from build123d import *

# Parameters (mm, degrees)
BOSS_EXTRUDE1_DEPTH = 9
SKETCH3_R           = 17.5
SKETCH3_R_2         = 7
SKETCH3_W           = 35
SKETCH3_H           = 9
BOSS_EXTRUDE2_DEPTH = 9


with BuildPart() as part:
    # Sketch1 → Boss-Extrude1 (new body)
    with BuildSketch(Plane.XY):
        with BuildLine():
            Line((0, -20), (86, -20))
            ThreePointArc((86, -20), (106, 0), (86, 20))
            Line((86, 20), (0, 20))
            Line((0, 20), (0, -20))
        make_face()
        with BuildLine():
            Line((63, 7), (86, 7))
            ThreePointArc((86, 7), (93, 0), (86, -7))
            Line((86, -7), (63, -7))
            ThreePointArc((63, -7), (56, 0), (63, 7))
        make_face(mode=Mode.SUBTRACT)
    extrude(amount=BOSS_EXTRUDE1_DEPTH)

    # Sketch3 → Boss-Extrude2 (add)
    with BuildSketch(Plane.XZ.offset(20)):
        with BuildLine():
            Line((0, 38), (0, 9))
            Line((0, 9), (35, 9))
            Line((35, 9), (35, 38))
            ThreePointArc((35, 38), (17.5, 20.5), (0, 38))
        make_face()
        with Locations((17.5, 38)):
            Circle(SKETCH3_R)
        with Locations((17.5, 38)):
            Circle(SKETCH3_R_2, mode=Mode.SUBTRACT)
        with Locations((17.5, 4.5)):
            Rectangle(SKETCH3_W, SKETCH3_H)
    boss_extrude2 = extrude(amount=-BOSS_EXTRUDE2_DEPTH)

    # Mirror1: Boss-Extrude2 across plane
    add(boss_extrude2.mirror(Plane.ZX))


solid = part.part
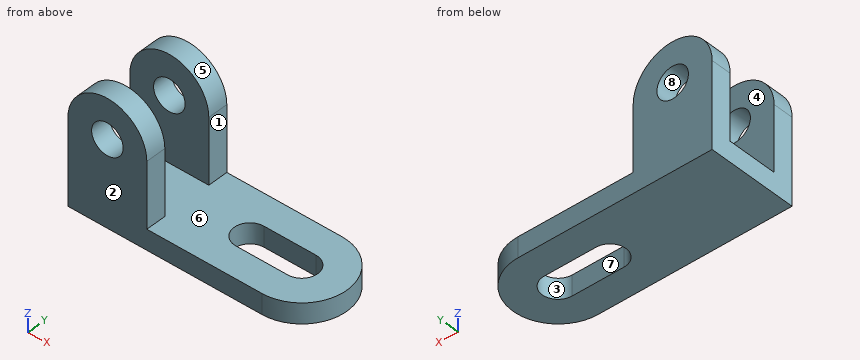
Model file for the job. Use its own axes, mm. Face numbers are marked on the shaded views. A direction names the side the tool comes from. Give positions to 0.01 mm unless a question says otherwise; leave off trailing zeros. Loops run counter-clockwise (first coordinate to the right, second up) from the corner with the lowest first, then second, coordinate; pieces in that order, holes last. Notation, with made-up numbers: (-40, 30.5) - (-30, 30.5) arc R27 ccw to (-30, 67.5) - close; hole circle Ø3 at (57.5, 25.25). An arc over 180 degrees is marked (long way). Use one line per item in the form item = value.
(1) Drop flat-ended pins along their axis: P1, Ø7, axis at y = -13.5, z = 19, coming from the +X side; P2, Ø8.5, axis at x = 17.5, z = 38, coming from the +Y side; P3, Ø2, axis at x = 64, y = -7.5, coming from the +Z side. Give the stop position or say it passes through.
Determined:
P1 = 35
P2 = through
P3 = 9
(2) Drill centre lines: L1, parallel to Y at x = 26, z = 42; L2, parallel to Z at x = 17, y = 15; L3, parallel to Z at x = 97, y = 0.5. Where is each one in solid material? Low to high.
Determined:
L1 = -20 to -11, 11 to 20
L2 = 0 to 31.02, 44.98 to 55.49
L3 = 0 to 9
(3) Pull direction X, two halves, no side cores. Call the marked faces 5, 6, 7 and 8: pulls with the +X half, pulls with the -X half, needs draft (parallel to the pull), parting line crosses it, or undercut.
Determined:
face_5 = parting line crosses it
face_6 = needs draft
face_7 = undercut
face_8 = undercut
(4) Cut at D-D (z = 6). Give the cut face in (x, y), then the cut area to 3 significant figures.
Determined:
outline = (0, -20) - (86, -20) arc R20 ccw to (86, 20) - (0, 20) - close; hole (63, -7) - (86, -7) arc R7 ccw to (86, 7) - (63, 7) arc R7 ccw to start
area = 3,590 mm^2
(5) 3-axis set-ups, long thin cutter, end or side, ignore diameter. For the marked faces 1, 2, 3 and 4: which of +Z, -Z, +X, -X, +Y, -Y reach the whole face in a straight line?
Determined:
face_1 = +Z, +X, +Y, -Y
face_2 = +Z, -Z, +X, -X, -Y
face_3 = +Z, -Z
face_4 = +Z, +X, -X
(6) Cut at A-A (z = 22.5). Give the cut face in (x, y).
Determined:
outline = (0, -20) - (35, -20) - (35, -11) - (0, -11) - close; (0, 11) - (35, 11) - (35, 20) - (0, 20) - close
(7) Cut at B-B (x = 17.5). Give the cut face in (y, z).
Determined:
outline = (-20, 0) - (20, 0) - (20, 31) - (11, 31) - (11, 9) - (-11, 9) - (-11, 31) - (-20, 31) - close; (-20, 45) - (-11, 45) - (-11, 55.5) - (-20, 55.5) - close; (11, 45) - (20, 45) - (20, 55.5) - (11, 55.5) - close
(8) Cut at C-C (y = 0). Give the cut face in (x, z), then the cut area to 3 significant figures.
Determined:
outline = (0, 0) - (56, 0) - (56, 9) - (0, 9) - close; (93, 0) - (106, 0) - (106, 9) - (93, 9) - close
area = 621 mm^2
